```python
from build123d import *

# Parameters (mm, degrees)
SKETCH3_W          = 5
SKETCH3_H          = 2.7
SKETCH4_W          = 5
SKETCH4_H          = 2.7
SKETCH5_W          = 5
SKETCH5_H          = 2.7
SKETCH6_W          = 5
SKETCH6_H          = 2.7
CUT_EXTRUDE1_DEPTH = 5


with BuildPart() as part:
    # Sketch1 → Revolve1 (revolve)
    with BuildSketch(Plane.XY):
        with BuildLine():
            Line((0, 0), (0, 21.5))
            Line((0, 21.5), (0.5, 22))
            Line((0.5, 22), (4.5, 22))
            Line((4.5, 22), (5, 21.5))
            Line((5, 21.5), (5, 11.5))
            ThreePointArc((5, 11.5), (5.146446609, 11.146446609), (5.5, 11))
            Line((5.5, 11), (29.5, 11))
            Line((29.5, 11), (30, 10.5))
            Line((30, 10.5), (30, 0))
            Line((30, 0), (0, 0))
        make_face()
    revolve(axis=Axis((30, 0, 0), (-1, 0, 0)))

    # Sketch2 → Cut-Revolve1 (revolve, cut)
    with BuildSketch(Plane.XY):
        Polygon((0, 0), (0, 6), (1, 5), (29, 5), (30, 6), (30, 0), align=None)
    revolve(axis=Axis((30, 0, 0), (-1, 0, 0)), mode=Mode.SUBTRACT)

    # Sketch3 → Cut-Revolve2 (revolve, cut)
    with BuildSketch(Plane.XY):
        with Locations((2.5, 16.85)):
            Rectangle(SKETCH3_W, SKETCH3_H)
    revolve(axis=Axis((5, 15.5, 0), (-1, 0, 0)), mode=Mode.SUBTRACT)

    # Sketch4 → Cut-Revolve3 (revolve, cut)
    with BuildSketch(Plane.XY.offset(15.5)):
        with Locations((2.5, 1.35)):
            Rectangle(SKETCH4_W, SKETCH4_H)
    revolve(axis=Axis((5, 0, 15.5), (-1, 0, 0)), mode=Mode.SUBTRACT)

    # Sketch5 → Cut-Revolve4 (revolve, cut)
    with BuildSketch(Plane.XY):
        with Locations((2.5, -14.15)):
            Rectangle(SKETCH5_W, SKETCH5_H)
    revolve(axis=Axis((5, -15.5, 0), (-1, 0, 0)), mode=Mode.SUBTRACT)

    # Sketch6 → Cut-Revolve5 (revolve, cut)
    with BuildSketch(Plane.XY.offset(-15.5)):
        with Locations((2.5, 1.35)):
            Rectangle(SKETCH6_W, SKETCH6_H)
    revolve(axis=Axis((5, 0, -15.5), (-1, 0, 0)), mode=Mode.SUBTRACT)

    # Sketch7 → Cut-Extrude1 (cut)
    with BuildSketch(Plane.ZY):
        with BuildLine():
            Line((11, 19.052558883), (11, -19.052558883))
            ThreePointArc((11, -19.052558883), (22, 0), (11, 19.052558883))
        make_face()
        with BuildLine():
            Line((-11, 19.052558883), (-11, -19.052558883))
            ThreePointArc((-11, -19.052558883), (-22, 0), (-11, 19.052558883))
        make_face()
    extrude(amount=-CUT_EXTRUDE1_DEPTH, mode=Mode.SUBTRACT)


solid = part.part
```
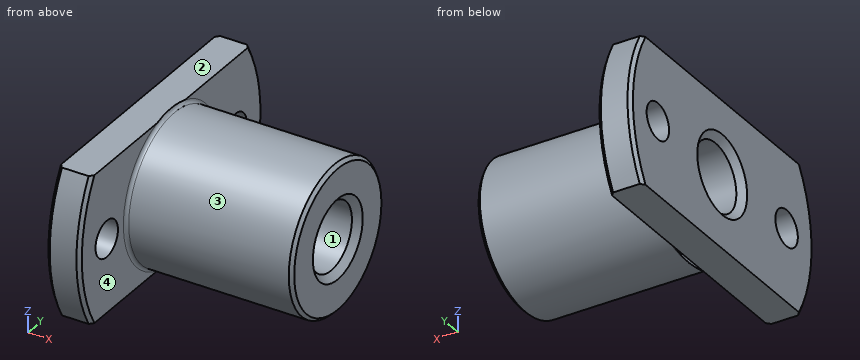
Verification items for the finished model (mm, model axes). Face numbers are marked on the shaded views. Coordinates: 2 decimals unless noted, no trailing zeros. Loops run counter-clockwise (first coordinate to the right, second up) from the corner with the lowest first, then second, coordinate; pieces in that order, holes last. Notation, with made-up numbers: (11, 72.25) - (36, 72.25) arc R17 ccw to (36, 85.25) - close; hole circle Ø3 at (-1.5, 84.5). An arc over 180 degrees is marked (long way). Put each result on its own line as item: value.
Item 1: Gauge pin test, flat ends, axial feed: pin 1 Ø3 at (x, z) = (4, -7) entering from -Y; pin 2 Ø1 at (y, z) = (-8.5, 3.5) entering from -X; pin 3 Ø8 at (x, y) = (11, 6) entering from -Z; pin 4 Ø8.5 at (y, z) = (15.5, 0) entering from +X. Record the tip position at first contact, or that the pin passes through.
Conclusion:
pin 1: stops at y = -21.3
pin 2: stops at x = 0
pin 3: stops at z = -10.82
pin 4: stops at x = 5.07
Item 2: Scan lines: line 1 along Y through (x, z) = (1.25, 0); line 2 along Z through (x, y) = (18.5, 0). Record each from-to range of solid material in increasing order.
Conclusion:
line 1: y = -22 to -18.2, -12.8 to -5, 5 to 12.8, 18.2 to 22
line 2: z = -11 to -5, 5 to 11
Item 3: Section check D-D (x = 10). Enter the section's corners in (y, z), then the cut area to 3 significant figures.
Conclusion:
outline: circle Ø22 at (0, 0); hole circle Ø10 at (0, 0)
area: 302 mm2
Item 4: Section check C-C (y = 0). Enter the section's corners in (x, z).
Conclusion:
outline: (0, -11) - (5, -11) - (5, -11.5) arc R0.5 cw to (5.5, -11) - (29.5, -11) - (30, -10.5) - (30, -6) - (29, -5) - (1, -5) - (0, -6) - close; (0, 6) - (1, 5) - (29, 5) - (30, 6) - (30, 10.5) - (29.5, 11) - (5.5, 11) arc R0.5 cw to (5, 11.5) - (5, 11) - (0, 11) - close
Item 5: Section check A-A (y = -15.5). Enter the section's corners in (x, z).
Conclusion:
outline: (0, -11) - (5, -11) - (5, -2.7) - (0, -2.7) - close; (0, 2.7) - (5, 2.7) - (5, 11) - (0, 11) - close
Item 6: Draft check along Z on the marked faces 1, 2, 3 and 4. Enter one of: pulls with the +Z half, pulls with the -Z half, needs draft (parallel to the pull), parting line crosses it, or undercut.
Conclusion:
face 1: undercut
face 2: pulls with the +Z half
face 3: parting line crosses it
face 4: needs draft
Item 7: Section check B-B (z = 0). Give the number of separate pieces and of enclosed holes in the cut face, then the cut area to 3 significant figures.
Conclusion:
separate pieces: 4
enclosed holes: 0
area: 413 mm2
